For this review, take the finished solid that the model builds, in its own axes (mm). Face numbers are marked on the shaded views. A direction names the side the tool comes from. Round coordinates to 2 decimals unless told otherwise and drop trailing zeros. Order: outer loops, then holes, each group sorted by start corner. A loop starts at its lowest first (then second) coordinate and runs counter-clockwise, first axis right, second up. Notation, with made-up numbers: M 26,17.5 L 72,17.5 A28 cw 72,44.5 Z; hole C -36,63.5 d4. An arc over 180 degrees is marked long. Use a Markdown table: item, result.
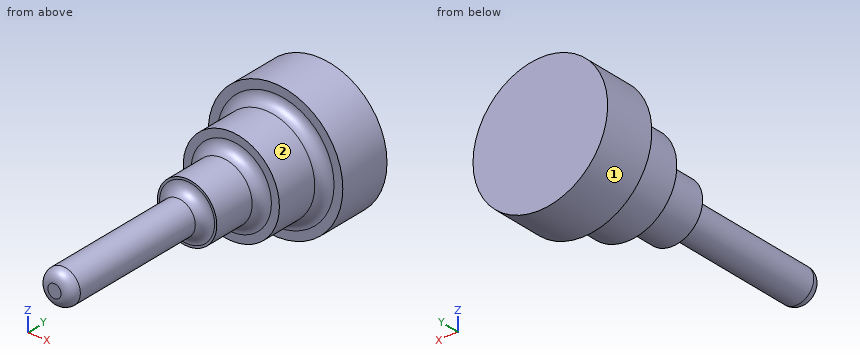
from build123d import *

# Parameters (mm, degrees)
F0_R     = 32.775689
F1_DEPTH = 25.4
F2_R     = 23.431872
F3_DEPTH = 25.4
F4_R     = 14.46384
F5_DEPTH = 25.4
F6_R     = 8.307558
F7_DEPTH = 76.2
F8_R     = 5.08


with BuildPart() as f1:
    # F0 (on Front) → F1 (new body)
    with BuildSketch(Plane.XZ):
        Circle(F0_R)
    extrude(amount=F1_DEPTH)

    # F2 (on face) → F3 (join)
    with BuildSketch(Plane.XZ.offset(25.4)):
        Circle(F2_R)
    extrude(amount=F3_DEPTH)

    # F4 (on face) → F5 (join)
    with BuildSketch(Plane.XZ.offset(50.8)):
        Circle(F4_R)
    extrude(amount=F5_DEPTH)

    # F6 (on face) → F7 (join)
    with BuildSketch(Plane.XZ.offset(76.2)):
        Circle(F6_R)
    extrude(amount=F7_DEPTH)

    # F8
    f8_edges = [f1.edges().sort_by_distance(p)[0] for p in [
        (-23.431872, -25.4, 0),
        (-14.46384, -50.8, 0),
        (-8.307558, -76.2, 0),
        (-8.307558, -152.4, 0),
    ]]
    fillet(f8_edges, radius=F8_R)


solid = f1.part
Q1. Add section A-A (y = -67). Write out the cut boundary in (x, z), then the cut area to 3 significant figures.
Determined:
| item | result |
|---|---|
| outline | C 0,0 d28.93 |
| area | 657 mm^2 |
Q2. Wall thickness on line 1 along Y through (x, z) = (30.5, 0); line 2 along Y through (x, z) = (3, -13); line 3 along X through (y, z) = (-10, 1): over which ranges is each line inside the solid? List them lowest first. Write a range as [from, to].
Determined:
| item | result |
|---|---|
| line 1 | y = [-25.4, 0] |
| line 2 | y = [-76.2, 0] |
| line 3 | x = [-32.76, 32.76] |
Q3. Clearance check with flat-ended pins moving along their axes: pin 1 (6 mm diameter, centred on x = -21.5, y = -31.5, fed in from -Z); pin 2 (4 mm diameter, centred on x = -21, z = 12.5, fed in from -Y); pin 3 (5 mm diameter, centred on x = 23.5, z = -15.5, fed in from -Y). State where each tip first meets the part, or that it passes through.
Determined:
| item | result |
|---|---|
| pin 1 | stops at z = -14.38 |
| pin 2 | stops at y = -50.8 |
| pin 3 | stops at y = -26.28 |
Q4. Machinability: for the marked faces 1 and 2, which of the approach directions +Z, -Z, +X, -X, +Y, -Y give a long, thin tool a straight path to every point of the face, cutting with its end or side? Answer none if there is none.
Determined:
| item | result |
|---|---|
| face 1 | +Y, -Y |
| face 2 | -Y |
Q5. Add section B-B (y = -44.5). Write out the cut boundary in (x, z), then the cut area to 3 significant figures.
Determined:
| item | result |
|---|---|
| outline | C 0,0 d46.86 |
| area | 1,720 mm^2 |
